Model file for the job. Use its own axes, mm. Face numbers are marked on the shaded views. A direction names the side the tool comes from. Round coordinates to 2 decimals unless told otherwise and drop trailing zeros. Write each loop counter-clockwise with the first axis right and the second up, starting at its lowest first coordinate (ties: lowest second). Pieces come first, ordered by that corner, then holes.
```python
from build123d import *

# Parameters (mm, degrees)
EXTRUDE004_DEPTH      = 20
EXTRUDE001_DEPTH      = 5
SKETCH002_R           = 57.15
SKETCH002_R_2         = 47.15
EXTRUDE002_DEPTH      = 270
EXTRUDE003_DEPTH      = 5
CLONE_PLACEMENT_ANGLE = 180
SKETCH_W              = 300
SKETCH_H              = 160
SKETCH_R              = 9
EXTRUDE_DEPTH         = 30
FILLET_R              = 1


with BuildPart() as lastplatte:
    # Sketch004 (on Face26 of Fusion) → Extrude004 (new body)
    with BuildSketch(Plane.XY.offset(300)):
        Polygon((65, 37.527767), (0, 75.055535), (-65, 37.527767), (-65, -37.527767), (0, -75.055535), (65, -37.527767), align=None)
    extrude(amount=-EXTRUDE004_DEPTH)


with BuildPart() as obj1:
    # Sketch001 → Extrude001 (new body, symmetric)
    with BuildSketch(Plane.XZ):
        Polygon((150, 30), (-150, 30), (-150, 80), (-100, 130), (100, 130), (150, 80), align=None)
    extrude(amount=EXTRUDE001_DEPTH, both=True)


with BuildPart() as obj2:
    # Sketch002 (on Face10 of Extrude) → Extrude002 (new body)
    with BuildSketch(Plane.XY.offset(30)):
        Circle(SKETCH002_R)
        Circle(SKETCH002_R_2, mode=Mode.SUBTRACT)
    extrude(amount=EXTRUDE002_DEPTH)


with BuildPart() as obj3:
    # Sketch003 → Extrude003 (new body, symmetric)
    with BuildSketch(Plane.YZ):
        Polygon((-80, 30), (-80, 80), (-65, 130), (-5, 130), (-5, 30), align=None)
    extrude(amount=EXTRUDE003_DEPTH, both=True)


with BuildPart() as obj4:
    # Clone base: copy of obj3
    add(obj3.part)


with BuildPart() as obj4_1:
    # Clone placement: moved
    add(obj4.part.rotate(Axis((0, 0, 0), (0, 0, 1)), CLONE_PLACEMENT_ANGLE))


with BuildPart() as fillet_body:
    # Sketch → Extrude (new body)
    with BuildSketch(Plane.XY):
        Rectangle(SKETCH_W, SKETCH_H)
        with Locations((-120, 50)):
            Circle(SKETCH_R, mode=Mode.SUBTRACT)
        with Locations((120, 50)):
            Circle(SKETCH_R, mode=Mode.SUBTRACT)
        with Locations((120, -50)):
            Circle(SKETCH_R, mode=Mode.SUBTRACT)
        with Locations((-120, -50)):
            Circle(SKETCH_R, mode=Mode.SUBTRACT)
    extrude(amount=EXTRUDE_DEPTH)

    # Fusion: union obj1, obj2, obj3, obj4
    add(obj1.part)
    add(obj2.part)
    add(obj3.part)
    add(obj4_1.part)

    # Fusion001: union lastplatte
    add(lastplatte.part)

    # Fillet
    fillet_edges = [fillet_body.edges().sort_by_distance(p)[0] for p in [
        (-57.15, 0, 130),
    ]]
    fillet(fillet_edges, radius=FILLET_R)


solid = fillet_body.part
```
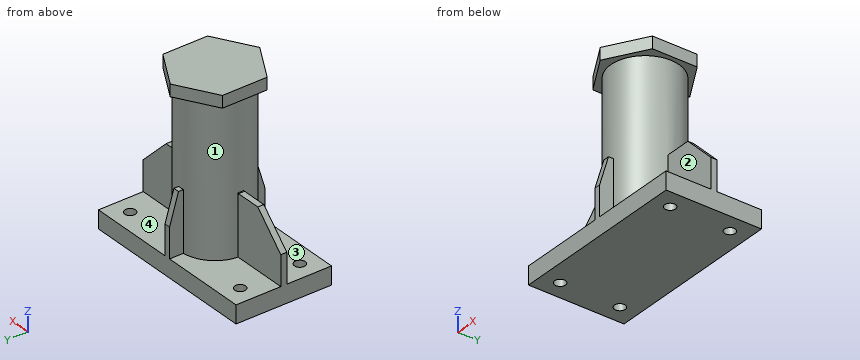
1) Which spindle directions (+Z, -Z, +X, -X, +Y, -Y) get a long thin tool onto all of the face, cutting with end or side? Do the marked faces 1, 2, 3 and 4. Say none if no direction does.
2) Cut at C-C on y = 0. List the corners of the cut face in (x, z), and give its area (3 significant figures).
3) Cut at D-D on x = 75. List the corners of the cut face in (y, z), and give its area (3 significant figures).
4) Cut at A-A on z = 71.5. List the corners of the cut face in (x, y).
5) Wall check: probe 1 along Y at (x, z) = (120, 9.25); probe 2 along X at (y, z) = (5.5, 122.5); probe 3 along Z at (x, y) = (0, -41). Give the ranges that are in metal, low to high.
6) Cut at B-B on x = 120. List the corners of the cut face in (y, z), and give its area (3 significant figures).
7) Flat gauge pins, fed straight in: pin 1 Ø11.5 at (y, z) = (71.5, 81.5) entering from +X; pin 2 Ø12.5 at (x, z) = (36, 56.5) entering from +Y; pin 3 Ø5 at (x, y) = (6, -8) entering from -Z; pin 4 Ø22.5 at (x, y) = (-84, -27) entering from +Z. Where does each tip first touch, or does it go through?
Result sheet:
1. face 1: none
1. face 2: +X, -Y
1. face 3: -X, -Y
1. face 4: +X, +Y
2. outline: (-150, 0) - (150, 0) - (150, 80) - (100, 130) - (57.15, 130) - (57.15, 280) - (65, 280) - (65, 300) - (-65, 300) - (-65, 280) - (-57.15, 280) - (-57.15, 131) arc R1 cw to (-58.15, 130) - (-100, 130) - (-150, 80) - close; hole (-47.15, 130) - (47.15, 130) - (47.15, 280) - (-47.15, 280) - close
2. area: 42,100 mm2
3. outline: (-80, 0) - (80, 0) - (80, 30) - (5, 30) - (5, 130) - (-5, 130) - (-5, 30) - (-80, 30) - close
3. area: 5,800 mm2
4. outline: (-150, -5) - (-56.93, -5) arc R57.15 ccw to (-5, -56.93) - (-5, -80) - (5, -80) - (5, -56.93) arc R57.15 ccw to (56.93, -5) - (150, -5) - (150, 5) - (56.93, 5) arc R57.15 ccw to (5, 56.93) - (5, 80) - (-5, 80) - (-5, 56.93) arc R57.15 ccw to (-56.93, 5) - (-150, 5) - close; hole (-46.88, -5) arc R47.15 ccw to (-5, -46.88) - (-5, -5) - close; hole (-46.88, 5) - (-5, 5) - (-5, 46.88) arc R47.15 ccw to start; hole (5, -46.88) arc R47.15 ccw to (46.88, -5) - (5, -5) - close; hole (5, 5) - (46.88, 5) arc R47.15 ccw to (5, 46.88) - close
5. probe 1: y = -80 to -59, -41 to 41, 59 to 80
5. probe 2: x = -56.88 to -46.83, -5 to 5, 46.83 to 56.88
5. probe 3: z = 0 to 130, 280 to 300
6. outline: (-80, 0) - (-59, 0) - (-59, 30) - (-80, 30) - close; (-41, 0) - (41, 0) - (41, 30) - (5, 30) - (5, 110) - (-5, 110) - (-5, 30) - (-41, 30) - close; (59, 0) - (80, 0) - (80, 30) - (59, 30) - close
6. area: 4,520 mm2
7. pin 1: stops at x = 5
7. pin 2: stops at y = 48.8
7. pin 3: stops at z = 0
7. pin 4: stops at z = 30
